Job drawing, mm, ordinate dimensions from the low corner. One solid piece. A direction names the side the tool comes from. Coordinates: 2 decimals unless noted, no trailing zeros. Write each loop counter-clockwise with the first axis right and the second up, starting at its lowest first coordinate (ties: lowest second). Pieces come first, ordered by that corner, then holes. Notation, with made-up numbers: M 13,-23 L 61,-23 A21 ccw 61,-4 Z; hole C 54.25,43.5 d11. An arc over 180 degrees is marked long. Answer as CSV lines item,"result". Start each with the question number.
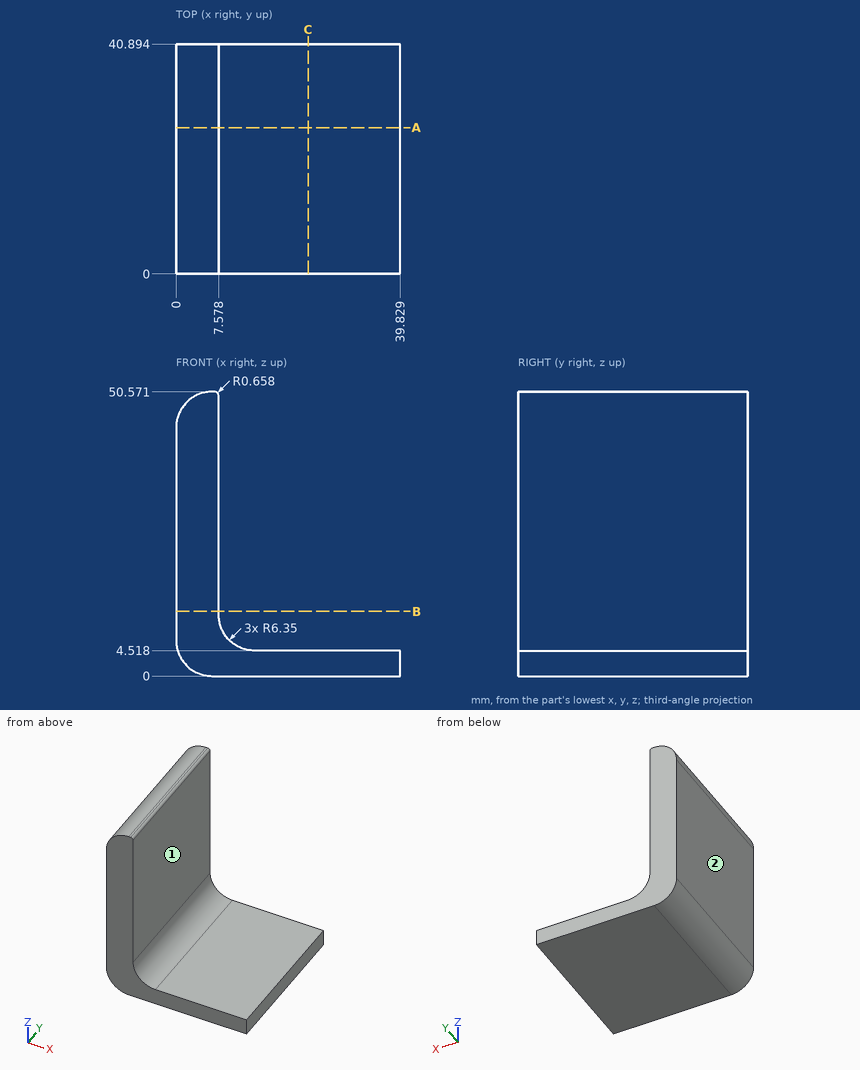
1) Band-saw the part on C-C, the plane x = 23.5. List the corners of the cut face in (y, z), plus the area to 3 significant figures.
2) Probe L1, parallel to Z at x = 20, y = 30.5; L2, parallel to X at y = 6, z = 39.5; L3, parallel to X at y = 22, z = 46.5. List the from-to ranges inside material, lowest first. Write a range as [from, to].
3) Band-saw the part on A-A, the plane y = 26. List the corners of the cut face in (x, z).
4) Pin check, flat tips, straight feed: P1, Ø10, axis at y = 32, z = 21, coming from the +X side; P2, Ø13, axis at x = 29, y = 23, coming from the +Z side; P3, Ø1, axis at x = 10, z = 8.5, coming from the +Y side. Stop position of each tip, or through.
5) Band-saw the part on B-B, the plane z = 11.5. List the corners of the cut face in (x, y), plus the area to 3 significant figures.
6) Tool access for the marked faces 1 and 2: list every direction of +Z, -Z, +X, -X, +Y, -Y with a clear straight run to the whole face (end or side of a thin tool).
Result sheet:
1,outline,"M 0,0 L 40.89,0 L 40.89,4.52 L 0,4.52 Z"
1,area,"185 mm²"
2,L1,"z = [0, 4.52]"
2,L2,"x = [0, 7.58]"
2,L3,"x = [0.42, 7.58]"
3,outline,"M 0,6.35 A6.35 ccw 6.35,0 L 39.83,0 L 39.83,4.52 L 13.93,4.52 A6.35 cw 7.58,10.87 L 7.58,49.91 A0.66 ccw 6.92,50.57 L 6.35,50.57 A6.35 ccw 0,44.22 Z"
4,P1,"stops at x = 7.58"
4,P2,"stops at z = 4.52"
4,P3,"passes through"
5,outline,"M 0,0 L 7.58,0 L 7.58,40.89 L 0,40.89 Z"
5,area,"310 mm²"
6,face 1,"+Z, +X, +Y, -Y"
6,face 2,"+Z, -Z, -X, +Y, -Y"
